from build123d import *

# Parameters (mm, degrees)
BOSS_EXTRUDE1_DEPTH                           = 9.5
CBORE_FOR_M12_HEX_HEAD_CAP_SCREW1_D           = 6.75
CBORE_FOR_M12_HEX_HEAD_CAP_SCREW1_DEPTH       = 16.51
CBORE_FOR_M12_HEX_HEAD_CAP_SCREW1_CBORE_D     = 25
CBORE_FOR_M12_HEX_HEAD_CAP_SCREW1_CBORE_DEPTH = 5
CBORE_FOR_M12_HEX_HEAD_CAP_SCREW1_TIP         = 2.027904589


with BuildPart() as part:
    # Sketch1 → Boss-Extrude1 (new, symmetric)
    with BuildSketch(Plane(origin=(0, 0, 0), x_dir=(0, 0, -1), z_dir=(1, 0, 0))):
        with BuildLine():
            Line((12.7, 0), (25.4, 0))
            Line((25.4, 0), (25.4, 19))
            Line((25.4, 19), (-25.4, 19))
            Line((-25.4, 19), (-25.4, 0))
            Line((-25.4, 0), (-12.7, 0))
            ThreePointArc((-12.7, 0), (0, 12.7), (12.7, 0))
        make_face()
    extrude(amount=BOSS_EXTRUDE1_DEPTH, both=True)

    # CBORE for M12 Hex Head Cap Screw1
    with Locations(Plane(origin=(0, 19, 0), x_dir=(1, 0, 0), z_dir=(0, 1, 0))):
        with Locations((0, 19.25446783), (0, -18.9082378)):
            CounterBoreHole(CBORE_FOR_M12_HEX_HEAD_CAP_SCREW1_D / 2, CBORE_FOR_M12_HEX_HEAD_CAP_SCREW1_CBORE_D / 2, CBORE_FOR_M12_HEX_HEAD_CAP_SCREW1_CBORE_DEPTH, depth=CBORE_FOR_M12_HEX_HEAD_CAP_SCREW1_DEPTH)
            with Locations((0, 0, -(CBORE_FOR_M12_HEX_HEAD_CAP_SCREW1_DEPTH + CBORE_FOR_M12_HEX_HEAD_CAP_SCREW1_TIP / 2))):  # 118° drill point
                Cone(0, CBORE_FOR_M12_HEX_HEAD_CAP_SCREW1_D / 2, CBORE_FOR_M12_HEX_HEAD_CAP_SCREW1_TIP, mode=Mode.SUBTRACT)


solid = part.part
Input: part model. Units: mm. Frame: model coordinates. A direction names the side the tool comes from. Coordinates: 2 decimals unless noted, no trailing zeros. Loops run counter-clockwise (first coordinate to the right, second up) from the corner with the lowest first, then second, coordinate; pieces in that order, holes last. Notation, with made-up numbers: (33.25, 54) -> (72.25, 54) arc R22 cw to (72.25, 60) -> close; hole circle Ø10 at (84.5, 17). An arc over 180 degrees is marked (long way). Write each question's results on one line, items separated by ' | '. Start each with the question number.
Q1. Section D-D, the plane x = 6.75. Return the cut outline in (y, z).
Q2. Pull-direction query (X, two-part tool) for faces 5 (the cylindrical face through (0.15, 16.54, 6.41)), 6 (the flat face through (9.5, 14, 0)), 7 (the flat face through (0, 19, 0)); classes: released by +X, released by -X, zero draft, split by the parting line, or undercut.
Q3. Section C-C, the plane y = 9.5. Return the cut outline in (x, z) (3 decimals).
Q4. Reachability of faces 1 (the cylindrical face through (0.133, 12.697, 0.279)), 2 (the cylindrical face through (-0.151, 16.535, -6.755)), 3 (the cylindrical face through (0.732, 8.164, 22.203)), 4 (the flat face through (-2, 14, 16)) from +Z, -Z, +X, -X, +Y, -Y: full face, straight path, thin tool, end or side. Return the list, or none.
Q5. Section B-B, the plane z = 9.5. Return the cut outline in (x, y).
Q6. Ray query, line 1 (Z direction, x = 0, y = 9.5); line 2 (Z direction, x = 0, y = 11.75); line 3 (Y direction, x = -3, z = 16). Return the intervals inside material, ascending. Write a range as from..to.
Q7. Section A-A, the plane y = 1.75. Return the cut outline in (x, z).
Q8. Pin query (flat end, axial travel): pin 1 (9.5 mm diameter, centred on x = -1.5, z = 12, fed in from +Y); pin 2 (5 mm diameter, centred on x = -3.5, y = 17, fed in from -Z). Return the tip coordinate at first contact, or that it passes through.
Found:
1) outline: (0, -25.4) -> (14, -25.4) -> (14, -8.73) -> (19, -8.73) -> (19, 8.39) -> (14, 8.39) -> (14, 25.4) -> (0, 25.4) -> (0, 12.7) arc R12.7 cw to (0, -12.7) -> close
2) face 5: undercut | face 6: released by +X | face 7: zero draft
3) outline: (-9.5, -25.4) -> (9.5, -25.4) -> (9.5, -8.429) -> (-9.5, -8.429) -> close; (-9.5, 8.429) -> (9.5, 8.429) -> (9.5, 25.4) -> (-9.5, 25.4) -> close; hole circle Ø6.75 at (0, -19.254); hole circle Ø6.75 at (0, 18.908)
4) face 1: +X, -X, -Y | face 2: -Z, +Y | face 3: +Y | face 4: +Z, +Y
5) outline: (-9.5, 8.43) -> (9.5, 8.43) -> (9.5, 19) -> (8.23, 19) -> (8.23, 14) -> (-8.23, 14) -> (-8.23, 19) -> (-9.5, 19) -> close
6) line 1: -25.4..-22.63, -15.88..-8.43, 8.43..15.53, 22.28..25.4 | line 2: -25.4..-22.63, -15.88..-4.82, 4.82..15.53, 22.28..25.4 | line 3: 0..14
7) outline: (-9.5, -25.4) -> (9.5, -25.4) -> (9.5, -12.58) -> (-9.5, -12.58) -> close; (-9.5, 12.58) -> (9.5, 12.58) -> (9.5, 25.4) -> (-9.5, 25.4) -> close; hole circle Ø4.29 at (0, -19.25); hole circle Ø4.29 at (0, 18.91)
8) pin 1: y = 14 | pin 2: z = -8.29
